The model under review builds one solid part; all positions refer to its coordinate system, in mm. Round coordinates to 2 decimals unless told otherwise and drop trailing zeros. Loops run counter-clockwise (first coordinate to the right, second up) from the corner with the lowest first, then second, coordinate; pieces in that order, holes last. Notation, with made-up numbers: (39, 32.25) -> (84, 32.25) arc R28 ccw to (84, 55.25) -> close; hole circle Ø10 at (17, 68). An arc over 180 degrees is marked (long way). Use a Markdown table: item, result. Add a question column.
1) Mouldability with a two-part tool opening along X and no side actions: class faces 1 (the flat face through (-11.05, 30, 2)), 2 (the flat face through (0, 0, -2)), 3 (the cylindrical face through (-0.243, 24.953, 2.367)) as released by +X, released by -X, zero draft, split by the parting line, or undercut.
2) Consider section A-A on y = 33. Give the boundary of the cut face in (x, z), plus the area to 3 significant figures.
3) Insertion check: pin 1 (4 mm diameter, centred on x = 5.52, y = 17.96, fed in from -Z); pin 2 (0.5 mm diameter, centred on y = 24.5, z = -8, fed in from -X); pin 3 (3 mm diameter, centred on x = 7.5, z = 15, fed in from +Y). Each pin has a flat end and moves straight along its axis. Give the tip position at first contact, or say it passes through.
4) Consider section B-B on z = 50.5. Give the boundary of the cut face in (x, y).
5) Wall thickness on probe 1 along Z at (x, y) = (0.5, 10); probe 2 along X at (y, z) = (24.5, -37); probe 3 along X at (y, z) = (32, 74.5): over which ranges is each line inside the solid? List them lowest first.
from build123d import *

# Parameters (mm, degrees)
SKETCH1_W             = 22.1
SKETCH1_H             = 338.1
BOSS_EXTRUDE1_DEPTH   = 36
CUT_EXTRUDE1_REACH    = 342.191
SKETCH2_R             = 11.05
SKETCH3_R             = 11.05
CUT_EXTRUDE2_DEPTH    = 175.247847906
F_5_0MM_DOWEL_HOLE4_D = 5
SKETCH16_W            = 4
SKETCH16_H            = 1
CUT_EXTRUDE3_DEPTH    = 341.190700196
SKETCH19_R            = 2.5
CUT_EXTRUDE4_DEPTH    = 10


with BuildPart() as part:
    # Sketch1 → Boss-Extrude1 (new body)
    with BuildSketch(Plane(origin=(0, 0, 0), x_dir=(1, 0, 0), z_dir=(0, 1, 0))):
        Rectangle(SKETCH1_W, SKETCH1_H)
    extrude(amount=BOSS_EXTRUDE1_DEPTH)

    # Sketch2 → Cut-Extrude1 (cut, up to next)
    with BuildSketch(Plane.XY.offset(169.05), mode=Mode.PRIVATE) as cut_extrude1_sk1:
        with Locations((0, 36)):
            Circle(SKETCH2_R)
    cut_extrude1_tool1 = extrude(cut_extrude1_sk1.sketch, amount=-CUT_EXTRUDE1_REACH, mode=Mode.PRIVATE) & part.part
    add(cut_extrude1_tool1.solids().sort_by_distance((0, 36, 169.05))[0], mode=Mode.SUBTRACT)

    # Sketch3 → Cut-Extrude2 (cut, through all)
    with BuildSketch(Plane(origin=(11.05, 0, 0), x_dir=(0, 0, -1), z_dir=(1, 0, 0))):
        with Locations((-169.05, 36)):
            Circle(SKETCH3_R)
        with Locations((169.05, 36)):
            Circle(SKETCH3_R)
    extrude(amount=-CUT_EXTRUDE2_DEPTH, mode=Mode.SUBTRACT)

    # Ø5.0mm Dowel Hole4 (through all)
    with Locations(Plane(origin=(11.05, 0, 0), x_dir=(0, 0, -1), z_dir=(1, 0, 0))):
        with Locations((-80, 8.94), (0, 8.94), (80, 8.94)):
            Hole(F_5_0MM_DOWEL_HOLE4_D / 2)

    # Sketch16 → Cut-Extrude3 (cut, through all)
    with BuildSketch(Plane(origin=(0, 0, -169.05), x_dir=(-1, 0, 0), z_dir=(0, 0, -1))):
        with Locations((9.05, 24.45)):
            Rectangle(SKETCH16_W, SKETCH16_H)
    extrude(amount=-CUT_EXTRUDE3_DEPTH, mode=Mode.SUBTRACT)

    # Sketch19 → Cut-Extrude4 (cut)
    with BuildSketch(Plane(origin=(0, 0, -169.05), x_dir=(-1, 0, 0), z_dir=(0, 0, -1))):
        with Locations((-5.525, 17.9625)):
            Circle(SKETCH19_R)
        with Locations((5.525, 5.9875)):
            Circle(SKETCH19_R)
    extrude(amount=-CUT_EXTRUDE4_DEPTH, mode=Mode.SUBTRACT)


solid = part.part
Result set:
| question | item | result |
|---|---|---|
| 1 | face 1 | released by -X |
| 1 | face 2 | zero draft |
| 1 | face 3 | undercut |
| 2 | outline | (-11.05, -158.42) -> (-10.63, -158.42) -> (-10.63, 158.42) -> (-11.05, 158.42) -> close; (10.63, -158.42) -> (11.05, -158.42) -> (11.05, 158.42) -> (10.63, 158.42) -> close |
| 2 | area | 263 mm2 |
| 3 | pin 1 | z = -159.05 |
| 3 | pin 2 | x = -7.05 |
| 3 | pin 3 | y = 29.59 |
| 4 | outline | (-11.05, 0) -> (11.05, 0) -> (11.05, 36) arc R11.05 cw to (-11.05, 36) -> (-11.05, 24.95) -> (-7.05, 24.95) -> (-7.05, 23.95) -> (-11.05, 23.95) -> close |
| 5 | probe 1 | -169.05 to -82.26, -77.74 to -2.26, 2.26 to 77.74, 82.26 to 169.05 |
| 5 | probe 2 | -7.05 to 11.05 |
| 5 | probe 3 | -11.05 to -10.3, 10.3 to 11.05 |
